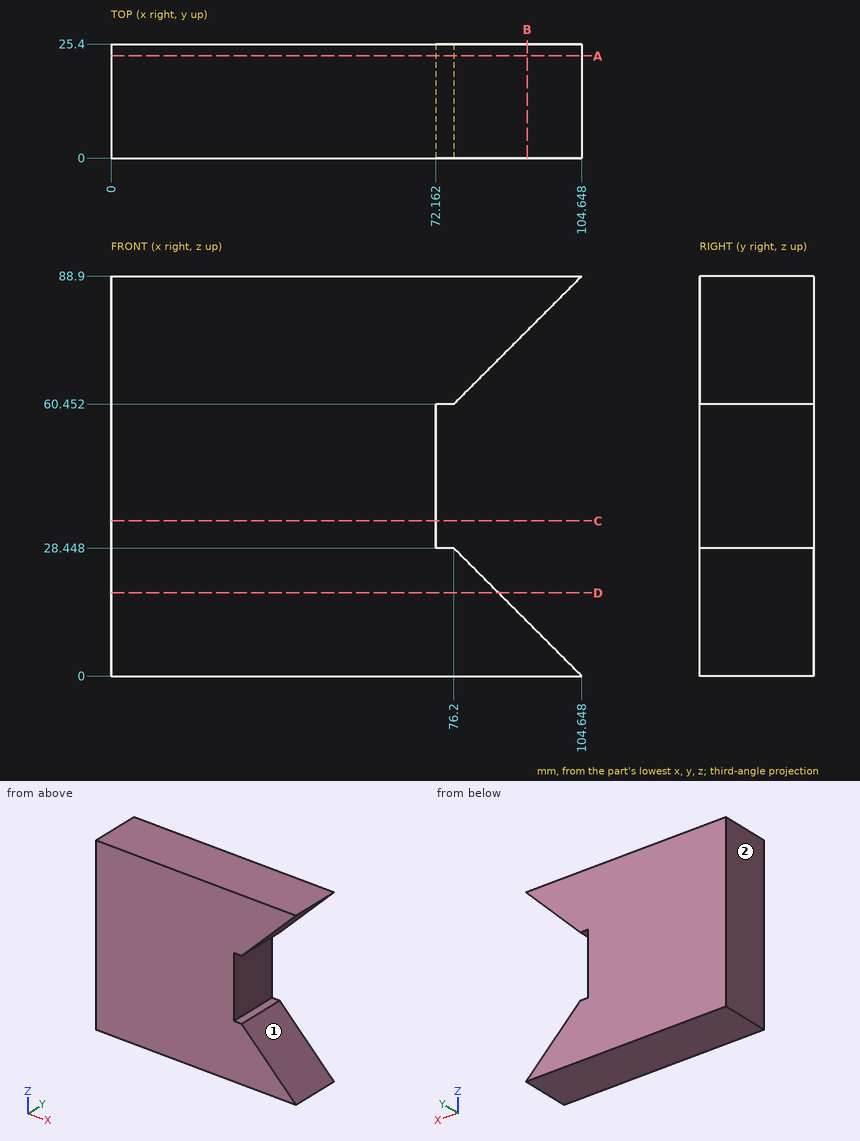
The figure shows three views and two pictorial views of one solid part (mm, origin at its lowest corner). Answer the questions. A direction names the side the tool comes from. Give positions to 0.01 mm unless a question says otherwise; leave off trailing zeros. Write each loop counter-clockwise with the first axis right and the second up, starting at its lowest first coordinate (ties: lowest second). Pieces come first, ordered by that corner, then holes.
Q1. The part is cut by section C-C on z = 34.5. Give the vertices of the cut face in (x, y), and give its area (3 significant figures).
Answer:
outline: (0, 0) - (72.16, 0) - (72.16, 25.4) - (0, 25.4) - close
area: 1,830 mm2
Q2. The part is cut by section B-B on x = 92.5. Give the vertices of the cut face in (y, z), and give its area (3 significant figures).
Answer:
outline: (0, 0) - (25.4, 0) - (25.4, 12.15) - (0, 12.15) - close; (0, 76.75) - (25.4, 76.75) - (25.4, 88.9) - (0, 88.9) - close
area: 617 mm2
Q3. The part is cut by section A-A on y = 22.75. Give the vertices of the cut face in (x, z).
Answer:
outline: (0, 0) - (104.65, 0) - (76.2, 28.45) - (72.16, 28.45) - (72.16, 60.45) - (76.2, 60.45) - (104.65, 88.9) - (0, 88.9) - close
Q4. Straight lines are drawn through the part: L1, parallel to Z at x = 73.5, y = 5.25; L2, parallel to X at y = 7.25, z = 39.5; L3, parallel to X at y = 23.25, z = 66. For each, find the intervals that lie inside material, in ascending order.
Answer:
L1: z = 0 to 28.45, 60.45 to 88.9
L2: x = 0 to 72.16
L3: x = 0 to 81.75
Q5. A tool of negligible diameter and unlimited length cuts with its end or side. For the marked faces 1 and 2, from which of +Z, -Z, +X, -X, +Y, -Y can it reach the whole face along a straight path? Write none if from no direction.
Answer:
face 1: +X, +Y, -Y
face 2: +Z, -Z, -X, +Y, -Y
Q6. The part is cut by section D-D on z = 18.5. Give the vertices of the cut face in (x, y), and give its area (3 significant figures).
Answer:
outline: (0, 0) - (86.15, 0) - (86.15, 25.4) - (0, 25.4) - close
area: 2,190 mm2
Q7. Given pin 1 (12.5 mm diameter, centred on y = 14.5, z = 37.5, fed in from +X); pin 2 (5 mm diameter, centred on y = 7.5, z = 11, fed in from +X), each flat-ended and moving along its own axis, determine where each tip first touches the part or whether it passes through.
Answer:
pin 1: stops at x = 72.16
pin 2: stops at x = 96.15
